from build123d import *

# Parameters (mm, degrees)
SKETCH1_R           = 23.8
SKETCH1_R_2         = 19
BOSS_EXTRUDE1_DEPTH = 80
SKETCH5_R           = 34.886960806
BOSS_EXTRUDE2_DEPTH = 25


with BuildPart() as part:
    # Sketch1 → Boss-Extrude1 (new body)
    with BuildSketch(Plane.XY):
        Circle(SKETCH1_R)
        Circle(SKETCH1_R_2, mode=Mode.SUBTRACT)
    extrude(amount=BOSS_EXTRUDE1_DEPTH)

    # Sketch5 → Boss-Extrude2 (add, symmetric)
    with BuildSketch(Plane(origin=(0, 0, 0), x_dir=(1, 0, 0), z_dir=(0, 1, 0))):
        with Locations((0, -102.473472637)):
            Circle(SKETCH5_R)
    extrude(amount=BOSS_EXTRUDE2_DEPTH, both=True)


solid = part.part
Here's how the part is built. I have some questions about the finished solid (model axes, mm). Coordinates: 2 decimals unless noted, no trailing zeros. Order: outer loops, then holes, each group sorted by start corner. A loop starts at its lowest first (then second) coordinate and runs counter-clockwise, first axis right, second up. Notation, with made-up numbers: (34, 71) - (44, 71) arc R21 cw to (44, 81) - close; hole circle Ø3 at (46.25, 9). An arc over 180 degrees is marked (long way). Use CSV: the item, a comma, the result in double quotes. Start each with the question number.
1. If we mould it in two halves opening along Y, with no side actions, what happens to faces 1 (the face through (-23.777, 1.046, 37.944)), 2 (the face through (18.12, 5.71, 36.09)), 3 (the face through (0.281, 0.266, 67.588)), 4 (the face through (0, 25, 102))? For each: +Y half, -Y half, draft (parallel to the pull), parting line (faces both ways), or undercut.
2. Suppose I cut it at C-C on z = 45. List the corners of the cut face in (x, y) for me, then the cut area to 3 significant figures.
3. Suppose I cut it at B-B on x = 0. List the corners of the cut face in (y, z) for me.
4. Suppose I cut it at A-A on y = 0. List the corners of the cut face in (x, z) for me, then the cut area to 3 significant figures.
5. Suppose I cut it at D-D on y = -9. List the corners of the cut face in (x, z) for me, then the cut area to 3 significant figures.
6. I'm going to push flat-ended pins straight in: pin 1 (4 mm diameter, centred on y = 13, z = 117, fed in from -X); pin 2 (12 mm diameter, centred on y = -5, z = 87, fed in from +X); pin 3 (2 mm diameter, centred on x = -27.5, y = -7, fed in from -Z); pin 4 (4 mm diameter, centred on x = -27.5, z = 37, fed in from +Y). Where does each tip first touch, or does it pass through?
7. Please list where these lines run through material, in increasing order: line 1 (Y direction, x = 0, z = 23); line 2 (X direction, y = -14, z = 43). Write a range as from..to.
Output:
1,face 1,"parting line"
1,face 2,"undercut"
1,face 3,"undercut"
1,face 4,"+Y half"
2,outline,"circle Ø47.6 at (0, 0); hole circle Ø38 at (0, 0)"
2,area,"645 mm2"
3,outline,"(-25, 67.59) - (-23.8, 67.59) - (-23.8, 0) - (-19, 0) - (-19, 67.59) - (19, 67.59) - (19, 0) - (23.8, 0) - (23.8, 67.59) - (25, 67.59) - (25, 137.36) - (-25, 137.36) - close"
4,outline,"(-23.8, 0) - (-19, 0) - (-19, 73.21) arc R34.89 ccw to (19, 73.21) - (19, 0) - (23.8, 0) - (23.8, 76.97) arc R34.89 ccw (long way) to (-23.8, 76.97) - close"
4,area,"4,540 mm2"
5,outline,"(-22.03, 0) - (-16.73, 0) - (-16.73, 71.86) arc R34.89 ccw to (16.73, 71.86) - (16.73, 0) - (22.03, 0) - (22.03, 75.42) arc R34.89 ccw (long way) to (-22.03, 75.42) - close"
5,area,"4,600 mm2"
6,pin 1,"stops at x = -32.56"
6,pin 2,"stops at x = 33.58"
6,pin 3,"stops at z = 79.78"
6,pin 4,"passes through"
7,line 1,"y = -23.8..-19, 19..23.8"
7,line 2,"x = -19.25..-12.85, 12.85..19.25"
